Model file for the job. Use its own axes, mm. A direction names the side the tool comes from. Round coordinates to 2 decimals unless told otherwise and drop trailing zeros. Loops run counter-clockwise (first coordinate to the right, second up) from the corner with the lowest first, then second, coordinate; pieces in that order, holes last. Notation, with made-up numbers: (-26.5, 41) -> (4.5, 41) arc R20 cw to (4.5, 48) -> close; hole circle Ø1 at (82, 39.25). An arc over 180 degrees is marked (long way). Use a Markdown table: item, result.
Autodesk Inventor part; units mm, degrees
ref_plane "YZ Plane" through (0, 0, 0) normal (1, 0, 0) x (0, 1, 0)
ref_plane "XZ Plane" through (0, 0, 0) normal (0, 1, 0) x (-1, 0, 0)
ref_plane "XY Plane" through (0, 0, 0) normal (0, 0, 1) x (1, 0, 0)
sketch "Sketch1" plane through (0, 0, 0) normal (0, 1, 0) x (-1, 0, 0)
  line L0 (0, 0) -> (30, 0)
  line L1 (30, 0) -> (30, -30)
  line L2 (30, -30) -> (0, -30)
  line L3 (0, -30) -> (0, 0)
  dimension "d0" = 30
  dimension "d1" = 30
extrude "Extrusion1" add sketch "Sketch1" along normal blind 2
sketch "Sketch2" plane through (0, 2, 0) normal (0, 1, 0) x (1, 0, 0)
  line L0 (-24.6588, 7.5) -> (-19.6588, 7.5)
  line L1 (-19.6588, 7.5) -> (-19.6588, 12.5)
  line L2 (-19.6588, 12.5) -> (-24.6588, 12.5)
  line L3 (-24.6588, 12.5) -> (-24.6588, 7.5)
  line L4 (-30, 0) -> (0, 0)
  line L5 (-24.6588, 17.5) -> (-19.6588, 17.5)
  line L6 (-19.6588, 17.5) -> (-19.6588, 22.5)
  line L7 (-19.6588, 22.5) -> (-24.6588, 22.5)
  line L8 (-24.6588, 22.5) -> (-24.6588, 17.5)
  line L9 (-10.1588, 7.5) -> (-5.1588, 7.5)
  line L10 (-5.1588, 7.5) -> (-5.1588, 22.5)
  line L11 (-5.1588, 22.5) -> (-10.1588, 22.5)
  line L12 (-10.1588, 22.5) -> (-10.1588, 7.5)
  dimension "d4" = 5
  dimension "d5" = 5
  dimension "d6" = 7.5
  dimension "d7" = 5
  dimension "d8" = 5
  dimension "d9" = 5
  dimension "d10" = 9.5
extrude "Extrusion2" cut sketch "Sketch2" against normal blind 2
sketch "Sketch3" plane through (0, 0, 0) normal (1, 0, 0) x (0, 0, -1)
  line L0 (30, 2) -> (0, 2)
  line L1 (30, 2) -> (0, 2)
  line L2 (0, 2) -> (0, -30)
  line L3 (0, -30) -> (30, -30)
  line L4 (30, -30) -> (30, 2)
  dimension "d15" = 32
extrude "Extrusion3" add sketch "Sketch3" along normal blind 2
properties part number "Head"
Q1. Band-saw the part on B-B, the plane z = -21. Give the cut face in (x, y).
Results list:
| item | result |
|---|---|
| outline | (-30, 0) -> (-24.66, 0) -> (-24.66, 2) -> (-30, 2) -> close; (-19.66, 0) -> (-10.16, 0) -> (-10.16, 2) -> (-19.66, 2) -> close; (-5.16, 0) -> (0, 0) -> (0, -30) -> (2, -30) -> (2, 2) -> (-5.16, 2) -> close |
Q2. Drill centre lines: L1, parallel to X at y = 0.5, z = -18.25; L2, parallel to Y at x = -14, z = -13. Where is each one in solid material? Low to high. Write a range as from..to.
Results list:
| item | result |
|---|---|
| L1 | x = -30..-24.66, -19.66..-10.16, -5.16..2 |
| L2 | y = 0..2 |
Q3. Tool access for faces 1 (the face through (-30, 1, -15)), 2 (the face through (-5.159, 1, -15)), 3 (the face through (0, -15, -15)): list every direction of +Z, -Z, +X, -X, +Y, -Y with a clear straight run to the whole face (end or side of a thin tool).
Results list:
| item | result |
|---|---|
| face 1 | +Z, -Z, -X, +Y, -Y |
| face 2 | +Y, -Y |
| face 3 | +Z, -Z, -X, -Y |
Q4. Pull direction X, two halves, no side cores. Call faces 4 (the face through (-15, 0, -15)), 5 (the face through (-8, 1, -7.5)), 6 (the face through (2, -14, -15)): released by +X, released by -X, zero draft, split by the parting line, or undercut.
Results list:
| item | result |
|---|---|
| face 4 | zero draft |
| face 5 | undercut |
| face 6 | released by +X |
Q5. Band-saw the part on C-C, the plane y = 0.5. Give the cut face in (x, z).
Results list:
| item | result |
|---|---|
| outline | (-30, -30) -> (2, -30) -> (2, 0) -> (-30, 0) -> close; hole (-24.66, -22.5) -> (-19.66, -22.5) -> (-19.66, -17.5) -> (-24.66, -17.5) -> close; hole (-24.66, -12.5) -> (-19.66, -12.5) -> (-19.66, -7.5) -> (-24.66, -7.5) -> close; hole (-10.16, -22.5) -> (-5.16, -22.5) -> (-5.16, -7.5) -> (-10.16, -7.5) -> close |
Q6. Band-saw the part on D-D, the plane y = -21. Give the cut face in (x, z), plus the area to 3 significant figures.
Results list:
| item | result |
|---|---|
| outline | (0, -30) -> (2, -30) -> (2, 0) -> (0, 0) -> close |
| area | 60.0 mm² |
Q7. Flat gauge pins, fed straight in: pin 1 (4 mm diameter, centred on x = -3, y = -5.5, fed in from -Z) (3 decimals); pin 2 (12 mm diameter, centred on x = -21.5, z = -26.5, fed in from -Y). Where does each tip first touch, or does it go through?
Results list:
| item | result |
|---|---|
| pin 1 | passes through |
| pin 2 | stops at y = 0 |
Q8. Band-saw the part on A-A, the plane x = -6. Give the cut face in (y, z).
Results list:
| item | result |
|---|---|
| outline | (0, -30) -> (2, -30) -> (2, -22.5) -> (0, -22.5) -> close; (0, -7.5) -> (2, -7.5) -> (2, 0) -> (0, 0) -> close |
